Here's how the part is built. I have some questions about the finished solid (model axes, mm). Face numbers are marked on the shaded views. A direction names the side the tool comes from. Round coordinates to 2 decimals unless told otherwise and drop trailing zeros. Write each loop counter-clockwise with the first axis right and the second up, starting at its lowest first coordinate (ties: lowest second). Pieces come first, ordered by that corner, then holes. Notation, with made-up numbers: (50.25, 78) - (74.25, 78) arc R24 cw to (74.25, 100) - close; hole circle Ø5 at (43, 21.25). An arc over 180 degrees is marked (long way). Use one line per item in the form item = value. Start each with the question number.
1. I want a section at B-B, the plane y = 3.75. List the corners of the cut face in (x, z) for me.
2. I want a section at C-C, the plane x = 0. List the corners of the cut face in (y, z) for me.
3. Which directions (+Z, -Z, +X, -X, +Y, -Y) give clear straight access to the entire face, cutting with the end or side of a thin tool? Please do the marked faces 4, 5, 6, 7 and 8.
4. I want a section at D-D, the plane y = 10.75. List the corners of the cut face in (x, z) for me, plus the area to 3 significant figures.
5. We'd pull the mould along Z, two halves only. Please class the marked faces 1, 2 and 3: +Z half, -Z half, draft (parallel to the pull), parting line (faces both ways), or undercut.
6. Will these pins go through, and if not, where does the flat tip stop? pin 1 (6 mm diameter, centred on x = -9.5, y = 17.5, fed in from +Z); pin 2 (1 mm diameter, centred on x = -16.5, z = -4, fed in from +Y); pin 3 (2 mm diameter, centred on y = 11.5, z = 12, fed in from -X).
7. I want a section at A-A, the plane z = 0. List the corners of the cut face in (x, y) for me, plus the area to 3 significant figures.
8. If I drill on line 1 along X through (y, z) = (3.5, 0); line 2 along Y through (x, z) = (5, 10.5); line 3 along Z through (x, y) = (-1, 3.75), over which ranges is the centre line in solid material (lowest first)?
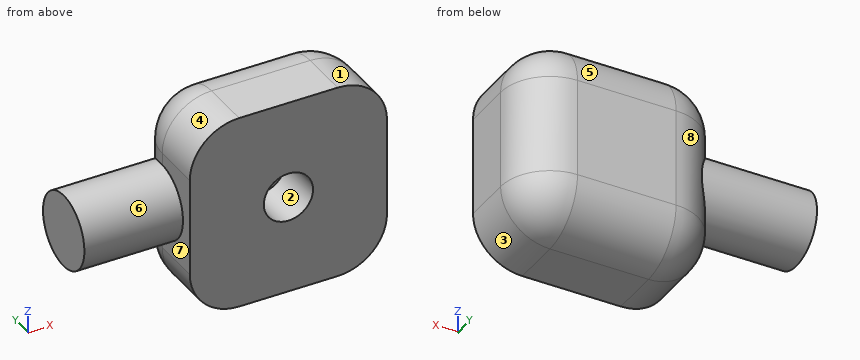
```python
from build123d import *

# Parameters (mm, degrees)
SKETCH1_W           = 40
SKETCH1_H           = 40
BOSS_EXTRUDE1_DEPTH = 20
SKETCH2_R           = 5
CUT_EXTRUDE1_DEPTH  = 10
SKETCH3_R           = 7.5
BOSS_EXTRUDE2_DEPTH = 20
FILLET1_R           = 10


with BuildPart() as part:
    # Sketch1 → Boss-Extrude1 (new body)
    with BuildSketch(Plane(origin=(0, 0, 0), x_dir=(1, 0, 0), z_dir=(0, 1, 0))):
        Rectangle(SKETCH1_W, SKETCH1_H)
    extrude(amount=BOSS_EXTRUDE1_DEPTH)

    # Sketch2 → Cut-Extrude1 (cut)
    with BuildSketch(Plane.XZ):
        with Locations(Location((0, 0, 0), (0, 0, 270))):
            Circle(SKETCH2_R)
    extrude(amount=-CUT_EXTRUDE1_DEPTH, mode=Mode.SUBTRACT)

    # Sketch3 → Boss-Extrude2 (add)
    with BuildSketch(Plane.ZY.offset(20)):
        with Locations((0, 10)):
            Circle(SKETCH3_R)
    extrude(amount=BOSS_EXTRUDE2_DEPTH)

    # Fillet1
    # the kernel refuses this fillet: 10 mm, written as the material it takes off along each edge
    with BuildSketch(Plane(origin=(10, 10, -10), x_dir=(0, 1, 0), z_dir=(1, 0, 0))) as fillet1_piece_1_section:
        Polygon((0, 0), (FILLET1_R, 0), (FILLET1_R, -FILLET1_R), (0, -FILLET1_R), align=None)
    fillet1_piece_1 = extrude(amount=FILLET1_R, mode=Mode.PRIVATE)
    fillet1_piece_1 = fillet1_piece_1 - Plane(origin=(10, 10, -10), x_dir=(0, -0.7071067811865475, 0.7071067811865475), z_dir=(1, 0, 0)) * Sphere(FILLET1_R, mode=Mode.PRIVATE)
    add(fillet1_piece_1, mode=Mode.SUBTRACT)
    with BuildSketch(Plane(origin=(10, 10, 10), x_dir=(1, 0, 0), z_dir=(0, 0, 1))) as fillet1_piece_2_section:
        Polygon((0, 0), (FILLET1_R, 0), (FILLET1_R, FILLET1_R), (0, FILLET1_R), align=None)
    fillet1_piece_2 = extrude(amount=FILLET1_R, mode=Mode.PRIVATE)
    fillet1_piece_2 = fillet1_piece_2 - Plane(origin=(10, 10, 10), x_dir=(-0.7071067811865475, -0.7071067811865475, 0), z_dir=(0, 0, 1)) * Sphere(FILLET1_R, mode=Mode.PRIVATE)
    add(fillet1_piece_2, mode=Mode.SUBTRACT)
    with BuildSketch(Plane(origin=(-10, 10, -10), x_dir=(0, 1, 0), z_dir=(-1, 0, 0))) as fillet1_piece_3_section:
        Polygon((0, 0), (FILLET1_R, 0), (FILLET1_R, FILLET1_R), (0, FILLET1_R), align=None)
    fillet1_piece_3 = extrude(amount=FILLET1_R, mode=Mode.PRIVATE)
    fillet1_piece_3 = fillet1_piece_3 - Plane(origin=(-10, 10, -10), x_dir=(0, -0.7071067811865475, 0.7071067811865475), z_dir=(-1, 0, 0)) * Sphere(FILLET1_R, mode=Mode.PRIVATE)
    add(fillet1_piece_3, mode=Mode.SUBTRACT)
    with BuildSketch(Plane(origin=(-10, 10, 10), x_dir=(-1, 0, 0), z_dir=(0, 0, 1))) as fillet1_piece_4_section:
        Polygon((0, 0), (FILLET1_R, 0), (FILLET1_R, -FILLET1_R), (0, -FILLET1_R), align=None)
    fillet1_piece_4 = extrude(amount=FILLET1_R, mode=Mode.PRIVATE)
    fillet1_piece_4 = fillet1_piece_4 - Plane(origin=(-10, 10, 10), x_dir=(0.7071067811865475, -0.7071067811865475, 0), z_dir=(0, 0, 1)) * Sphere(FILLET1_R, mode=Mode.PRIVATE)
    add(fillet1_piece_4, mode=Mode.SUBTRACT)
    with BuildSketch(Plane(origin=(20, 20, -10), x_dir=(0, -1, 0), z_dir=(0, 0, 1)), Plane(origin=(10, 20, 20), x_dir=(0, -1, 0), z_dir=(-1, 0, 0))) as fillet1_piece_5:
        with BuildLine():
            CenterArc((FILLET1_R, -FILLET1_R), FILLET1_R, 90, 90)
            Line((0, -FILLET1_R), (0, 0))
            Line((0, 0), (FILLET1_R, 0))
        make_face()
    extrude(amount=20, mode=Mode.SUBTRACT)
    with BuildSketch(Plane(origin=(-10, 20, -20), x_dir=(0, 0, 1), z_dir=(1, 0, 0))) as fillet1_piece_6:
        with BuildLine():
            CenterArc((FILLET1_R, FILLET1_R), FILLET1_R, 180, 90)
            Line((0, FILLET1_R), (0, 0))
            Line((0, 0), (FILLET1_R, 0))
        make_face()
    extrude(amount=20, mode=Mode.SUBTRACT)
    with BuildSketch(Plane(origin=(-20, 20, 10), x_dir=(0, -1, 0), z_dir=(0, 0, -1))) as fillet1_piece_7_section:
        with BuildLine():
            CenterArc((FILLET1_R, -FILLET1_R), FILLET1_R, 90, 90)
            Line((0, -FILLET1_R), (0, 0))
            Line((0, 0), (FILLET1_R, 0))
        make_face()
    fillet1_piece_7 = extrude(amount=20, mode=Mode.PRIVATE)
    fillet1_piece_7 = fillet1_piece_7 - Plane(origin=(-17.405135358, 10, 0), x_dir=(0, 0, 1), z_dir=(1, 0, 0)) * Cylinder(7.5, 80, mode=Mode.PRIVATE)
    add(fillet1_piece_7, mode=Mode.SUBTRACT)
    with BuildSketch(Plane(origin=(-20, -25, -20), x_dir=(0, 0, 1), z_dir=(0, 1, 0)), Plane(origin=(-20, -25, 20), x_dir=(1, 0, 0), z_dir=(0, 1, 0))) as fillet1_piece_8:
        with BuildLine():
            CenterArc((FILLET1_R, FILLET1_R), FILLET1_R, 180, 90)
            Line((0, FILLET1_R), (0, 0))
            Line((0, 0), (FILLET1_R, 0))
        make_face()
    extrude(amount=35, mode=Mode.SUBTRACT)
    with BuildSketch(Plane(origin=(20, -25, -20), x_dir=(0, 0, 1), z_dir=(0, 1, 0)), Plane(origin=(20, -25, 20), x_dir=(-1, 0, 0), z_dir=(0, 1, 0))) as fillet1_piece_9:
        with BuildLine():
            CenterArc((FILLET1_R, -FILLET1_R), FILLET1_R, 90, 90)
            Line((0, -FILLET1_R), (0, 0))
            Line((0, 0), (FILLET1_R, 0))
        make_face()
    extrude(amount=35, mode=Mode.SUBTRACT)


solid = part.part
```
Model answer:
q1.outline = (-40, -4.15) - (-20, -4.15) - (-20, -10) arc R10 ccw to (-10, -20) - (10, -20) arc R10 ccw to (20, -10) - (20, 10) arc R10 ccw to (10, 20) - (-10, 20) arc R10 ccw to (-20, 10) - (-20, 4.15) - (-40, 4.15) - close; hole circle Ø10 at (0, 0)
q2.outline = (0, -20) - (10, -20) arc R10 ccw to (20, -10) - (20, 10) arc R10 ccw to (10, 20) - (0, 20) - (0, 5) - (10, 5) - (10, -5) - (0, -5) - close
q3.face_4 = +Z, -X, +Y, -Y
q3.face_5 = +Z, +X, -X, +Y
q3.face_6 = -X
q3.face_7 = -X, -Y
q3.face_8 = -X, +Y
q4.outline = (-40, -7.46) - (-19.97, -7.46) - (-19.97, -10) arc R9.97 ccw to (-10, -19.97) - (10, -19.97) arc R9.97 ccw to (19.97, -10) - (19.97, 10) arc R9.97 ccw to (10, 19.97) - (-10, 19.97) arc R9.97 ccw to (-19.97, 10) - (-19.97, 7.46) - (-40, 7.46) - close
q4.area = 1,810 mm2
q5.face_1 = +Z half
q5.face_2 = undercut
q5.face_3 = -Z half
q6.pin_1 = 18.93
q6.pin_2 = 18
q6.pin_3 = -19.89
q7.outline = (-40, 2.5) - (-20, 2.5) - (-20, 0) - (-5, 0) - (-5, 10) - (5, 10) - (5, 0) - (20, 0) - (20, 10) arc R10 ccw to (10, 20) - (-10, 20) arc R10 ccw to (-16.61, 17.5) - (-40, 17.5) - close
q7.area = 965 mm2
q8.line_1 = -40 to -5, 5 to 20
q8.line_2 = 0 to 19.99
q8.line_3 = -20 to -4.9, 4.9 to 20
